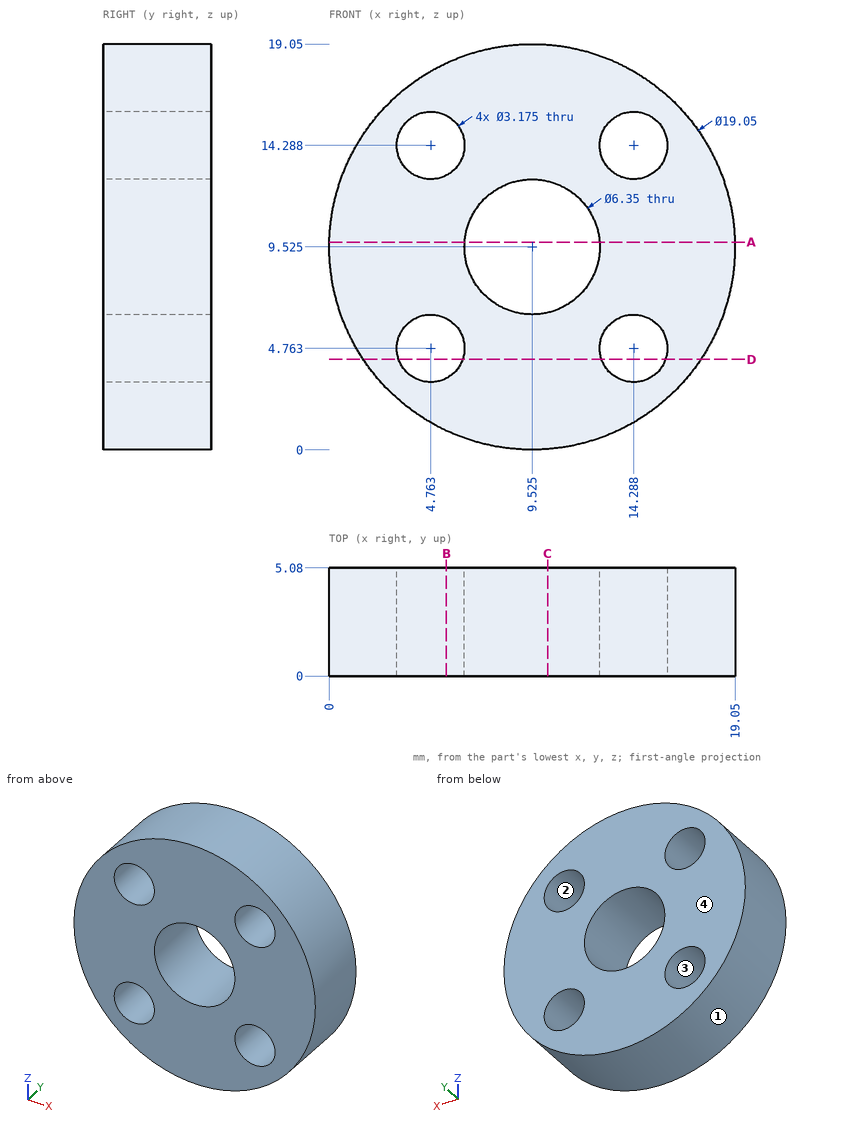
Design review of the part shown in the three views and the two pictorial views. Dimensions are in mm from the part's minimum x, y and z. Give positions to 0.01 mm unless a question says otherwise; leave off trailing zeros. Order: outer loops, then holes, each group sorted by start corner. A loop starts at its lowest first (then second) coordinate and runs counter-clockwise, first axis right, second up. Notation, with made-up numbers: (4.25, 12.25) -> (24.25, 12.25) arc R24 ccw to (24.25, 35.25) -> close; hole circle Ø10 at (-3.5, 7). An arc over 180 degrees is marked (long way). Write each question's results on one line, items separated by ' | '. Start each with the question number.
Q1. Mouldability with a two-part tool opening along Z and no side actions: class the marked faces 1, 2, 3 and 4 as +Z half, -Z half, draft (parallel to the pull), parting line (faces both ways), or undercut.
Q2. Add section B-B on x = 5.5. Give the boundary of the cut face in (y, z).
Q3. Wall thickness on L1, parallel to Z at x = 15.5, y = 4.7 (1 decimal); L2, parallel to X at y = 1.9, z = 13 (1 decimal); L3, parallel to X at y = 3.9, z = 15 (1 decimal): over which ranges is each line inside the solid? List them lowest first. Write a range as from..to.
Q4. Add section C-C on x = 10.25. Give the boundary of the cut face in (y, z).
Q5. Add section A-A on z = 9.75. Give the boundary of the cut face in (x, y).
Q6. For pin 1 (2 mm diameter, centred on y = 3, z = 4, fed in from +X), flat-tipped, find the tip position at first contact; note if it passes through.
Q7. Add section D-D on z = 4.25. Give the boundary of the cut face in (x, y) (1 decimal).
Found:
1) face 1: parting line | face 2: undercut | face 3: undercut | face 4: draft
2) outline: (0, 0.89) -> (5.08, 0.89) -> (5.08, 3.36) -> (0, 3.36) -> close; (0, 6.17) -> (5.08, 6.17) -> (5.08, 12.88) -> (0, 12.88) -> close; (0, 15.69) -> (5.08, 15.69) -> (5.08, 18.16) -> (0, 18.16) -> close
3) L1: z = 2.1..3.7, 5.8..13.3, 15.3..16.9 | L2: x = 0.7..3.8, 5.7..13.4, 15.2..18.4 | L3: x = 1.7..3.3, 6.2..12.9, 15.7..17.3
4) outline: (0, 0.03) -> (5.08, 0.03) -> (5.08, 6.43) -> (0, 6.43) -> close; (0, 12.62) -> (5.08, 12.62) -> (5.08, 19.02) -> (0, 19.02) -> close
5) outline: (0, 0) -> (6.36, 0) -> (6.36, 5.08) -> (0, 5.08) -> close; (12.69, 0) -> (19.05, 0) -> (19.05, 5.08) -> (12.69, 5.08) -> close
6) pin 1: stops at x = 17.91
7) outline: (1.6, 0) -> (3.3, 0) -> (3.3, 5.1) -> (1.6, 5.1) -> close; (6.3, 0) -> (12.8, 0) -> (12.8, 5.1) -> (6.3, 5.1) -> close; (15.8, 0) -> (17.5, 0) -> (17.5, 5.1) -> (15.8, 5.1) -> close
